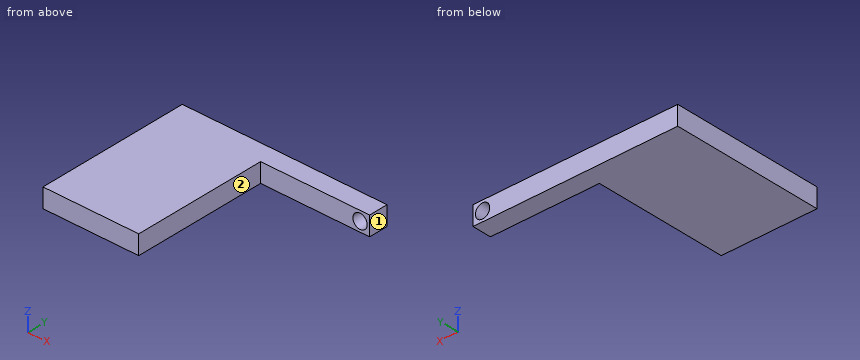
from build123d import *

# Parameters (mm, degrees)
BOSS_EXTRUDE1_DEPTH     = 10
CUT_EXTRUDE1_DEPTH      = 134.663857908
CUT_EXTRUDE1_DEPTH_BACK = 134.663857908
SKETCH2_R               = 3.735264888


with BuildPart() as part:
    # Sketch1 → Boss-Extrude1 (new body)
    with BuildSketch(Plane.XY):
        Polygon((0.330578512, 197.933884298), (0.330578512, 187.933884298), (-56.611570248, 187.933884298), (-56.611570248, 117.933884298), (-106.611570248, 117.933884298), (-106.611570248, 197.933884298), align=None)
    extrude(amount=BOSS_EXTRUDE1_DEPTH)

    # Sketch2 → Cut-Extrude1 (cut, two sides: drawn at the far end of the back side and taken through both)
    with BuildSketch(Plane(origin=(0, 197.933884298, 0), x_dir=(1, 0, 0), z_dir=(0, 1, 0)).offset(-CUT_EXTRUDE1_DEPTH_BACK)):
        with Locations(Location((-4.669421488, -5, 0), (0, 0, 180))):
            Circle(SKETCH2_R)
    extrude(amount=CUT_EXTRUDE1_DEPTH + CUT_EXTRUDE1_DEPTH_BACK, mode=Mode.SUBTRACT)


solid = part.part
Input: part model. Units: mm. Frame: model coordinates. Face numbers are marked on the shaded views. A direction names the side the tool comes from. Coordinates: 2 decimals unless noted, no trailing zeros. Order: outer loops, then holes, each group sorted by start corner. A loop starts at its lowest first (then second) coordinate and runs counter-clockwise, first axis right, second up. Notation, with made-up numbers: M -8,27.25 L 20,27.25 A21 cw 20,49.25 Z; hole C 74,40.5 d5. An arc over 180 degrees is marked long. One line per question, with ' | ' between items.
Item 1: Section A-A (z = 5). Output: boundary loops of the cut face in (x, y), then the cut area to 3 significant figures.
Geometry results:
outline: M -106.61,117.93 L -56.61,117.93 L -56.61,187.93 L -8.4,187.93 L -8.4,197.93 L -106.61,197.93 Z; M -0.93,187.93 L 0.33,187.93 L 0.33,197.93 L -0.93,197.93 Z | area: 4,490 mm^2
Item 2: Section B-B (x = -40). Output: boundary loops of the cut face in (y, z), then the cut area to 3 significant figures.
Geometry results:
outline: M 187.93,0 L 197.93,0 L 197.93,10 L 187.93,10 Z | area: 100 mm^2
Item 3: Section C-C (y = 175.5). Output: boundary loops of the cut face in (x, z), then the cut area to 3 significant figures.
Geometry results:
outline: M -106.61,0 L -56.61,0 L -56.61,10 L -106.61,10 Z | area: 500 mm^2
Item 4: Pin query (flat end, axial travel): pin 1 (6 mm diameter, centred on x = -52, z = 2, fed in from -Y); pin 2 (3 mm diameter, centred on y = 183, z = 8.5, fed in from +X). Return the tip coordinate at first contact, or that it passes through.
Geometry results:
pin 1: stops at y = 187.93 | pin 2: stops at x = -56.61
Item 5: Ray query, line 1 along X through (y, z) = (193, 5); line 2 along X through (y, z) = (185, 7.5). Return the intervals inside material, ascending.
Geometry results:
line 1: x = -106.61 to -8.4, -0.93 to 0.33 | line 2: x = -106.61 to -56.61
Item 6: Reachability of the marked faces 1 and 2 from +Z, -Z, +X, -X, +Y, -Y: full face, straight path, thin tool, end or side. Return the list, or none.
Geometry results:
face 1: +Z, -Z, +X, +Y, -Y | face 2: +Z, -Z, +X, -Y
